from build123d import *

# Parameters (mm, degrees)
SKETCH_2_W      = 70
SKETCH_2_H      = 20
SKETCH_2_R      = 2.6
EXTRUDE_1_DEPTH = 5
FILLET_1_R      = 5


with BuildPart() as part:
    # ｽｹｯﾁ2 → ﾎﾞｽ - 押し出し1 (new body)
    with BuildSketch(Plane.XY):
        with Locations((25, 0)):
            Rectangle(SKETCH_2_W, SKETCH_2_H)
        with Locations((25, 0)):
            Circle(SKETCH_2_R, mode=Mode.SUBTRACT)
        with Locations((50, 0)):
            Circle(SKETCH_2_R, mode=Mode.SUBTRACT)
        Circle(SKETCH_2_R, mode=Mode.SUBTRACT)
    extrude(amount=EXTRUDE_1_DEPTH)

    # ﾌｨﾚｯﾄ1
    fillet_1_edges = [part.edges().sort_by_distance(p)[0] for p in [
        (-10, 10, 2.5),
        (60, 10, 2.5),
        (60, -10, 2.5),
        (-10, -10, 2.5),
    ]]
    fillet(fillet_1_edges, radius=FILLET_1_R)


solid = part.part
Model file for the job. Use its own axes, mm. Give positions to 0.01 mm unless a question says otherwise; leave off trailing zeros. Order: outer loops, then holes, each group sorted by start corner. A loop starts at its lowest first (then second) coordinate and runs counter-clockwise, first axis right, second up. Notation, with made-up numbers: (43, -23) -> (60, -23) arc R21 cw to (60, -3) -> close; hole circle Ø9 at (42, 46.25). An arc over 180 degrees is marked (long way). Use CSV: the item, a comma, the result in double quotes.
1. Band-saw the part on B-B, the plane z = 2.45. Give the cut face in (x, y), then the cut area to 3 significant figures.
Outcome:
outline,"(-10, -5) arc R5 ccw to (-5, -10) -> (55, -10) arc R5 ccw to (60, -5) -> (60, 5) arc R5 ccw to (55, 10) -> (-5, 10) arc R5 ccw to (-10, 5) -> close; hole circle Ø5.2 at (0, 0); hole circle Ø5.2 at (25, 0); hole circle Ø5.2 at (50, 0)"
area,"1,310 mm²"
2. Band-saw the part on C-C, the plane y = 0. Give the cut face in (x, z), then the cut area to 3 significant figures.
Outcome:
outline,"(-10, 0) -> (-2.6, 0) -> (-2.6, 5) -> (-10, 5) -> close; (2.6, 0) -> (22.4, 0) -> (22.4, 5) -> (2.6, 5) -> close; (27.6, 0) -> (47.4, 0) -> (47.4, 5) -> (27.6, 5) -> close; (52.6, 0) -> (60, 0) -> (60, 5) -> (52.6, 5) -> close"
area,"272 mm²"
3. Drill centre lines: line 1 along X through (y, z) = (-0.25, 2.5); line 2 along Y through (x, z) = (0, 1.35); line 3 along Y through (x, z) = (-1.5, 0.6). Where is each one in solid material? Low to high. Write a range as from..to.
Outcome:
line 1,"-10..-2.59, 2.59..22.41, 27.59..47.41, 52.59..60"
line 2,"-10..-2.6, 2.6..10"
line 3,"-10..-2.12, 2.12..10"
4. Band-saw the part on A-A, the plane x = 1. Give the cut face in (y, z), then the cut area to 3 significant figures.
Outcome:
outline,"(-10, 0) -> (-2.4, 0) -> (-2.4, 5) -> (-10, 5) -> close; (2.4, 0) -> (10, 0) -> (10, 5) -> (2.4, 5) -> close"
area,"76.0 mm²"
5. Band-saw the part on D-D, the plane x = 50. Give the cut face in (y, z), then the cut area to 3 significant figures.
Outcome:
outline,"(-10, 0) -> (-2.6, 0) -> (-2.6, 5) -> (-10, 5) -> close; (2.6, 0) -> (10, 0) -> (10, 5) -> (2.6, 5) -> close"
area,"74.0 mm²"
6. Drop a flat-ended pin along its axis: pin 1 (2 mm diameter, centred on x = 27.5, y = 4, fed in from -Z). Give the stop position or say it passes through.
Outcome:
pin 1,"z = 0"
7. Mould opens along X. For faces 1 (the flat face through (25, -10, 2)), 2 (the cylindrical face through (-9, 8, 3)), 3 (the cylindrical face through (27.48, 0.78, 2.46)) say: +X half, -X half, draft (parallel to the pull), parting line (faces both ways), or undercut.
Outcome:
face 1,"draft"
face 2,"-X half"
face 3,"undercut"
